```python
from build123d import *

# Parameters (mm, degrees)
ESQUISSE1_W        = 12.8
ESQUISSE1_H        = 9
BOSS_EXTRU_1_DEPTH = 6.8
ESQUISSE2_W        = 1
ESQUISSE2_H        = 2
BOSS_EXTRU_2_DEPTH = 4
ESQUISSE3_R        = 3
BOSS_EXTRU_3_DEPTH = 9
ESQUISSE4_R        = 1.5
BOSS_EXTRU_4_DEPTH = 10


with BuildPart() as part:
    # Esquisse1 → Boss.-Extru.1 (new body)
    with BuildSketch(Plane.XY):
        with Locations((6.4, 4.5)):
            Rectangle(ESQUISSE1_W, ESQUISSE1_H)
    extrude(amount=BOSS_EXTRU_1_DEPTH)

    # Esquisse2 → Boss.-Extru.2 (add)
    with BuildSketch(Plane.XZ):
        with Locations((1.4, 2.9)):
            Rectangle(ESQUISSE2_W, ESQUISSE2_H)
        with Locations((6.4, 2.9)):
            Rectangle(ESQUISSE2_W, ESQUISSE2_H)
        with Locations((11.4, 2.9)):
            Rectangle(ESQUISSE2_W, ESQUISSE2_H)
    extrude(amount=BOSS_EXTRU_2_DEPTH)

    # Esquisse3 → Boss.-Extru.3 (add)
    with BuildSketch(Plane(origin=(0, 9, 0), x_dir=(1, 0, 0), z_dir=(0, 1, 0))):
        with Locations((6.4, -3.4)):
            Circle(ESQUISSE3_R)
    extrude(amount=BOSS_EXTRU_3_DEPTH)

    # Esquisse4 → Boss.-Extru.4 (add)
    with BuildSketch(Plane(origin=(0, 18, 0), x_dir=(1, 0, 0), z_dir=(0, 1, 0))):
        with Locations((6.4, -3.4)):
            Circle(ESQUISSE4_R)
    extrude(amount=BOSS_EXTRU_4_DEPTH)


solid = part.part
```
Source: CAD feature listing. Evaluate the final solid. Frame: model axes, mm. A direction names the side the tool comes from. Round coordinates to 2 decimals unless told otherwise and drop trailing zeros. Loops run counter-clockwise (first coordinate to the right, second up) from the corner with the lowest first, then second, coordinate; pieces in that order, holes last.
1. Mould query, pull axis X, two halves, no side actions, for faces 6 (the flat face through (1.4, -2, 1.9)), 7 (the cylindrical face through (3.4, 13.4, 3.3)), 8 (the flat face through (6.3, 0, 4.1)). Classes: released by +X, released by -X, zero draft, split by the parting line, or undercut.
2. Section query C-C on y = 13. Output: boundary loops of the cut face in (x, z), and give its area (3 significant figures).
3. Section query D-D on x = 6.4. Output: boundary loops of the cut face in (y, z).
4. Access query for faces 1 (the flat face through (0.9, -2, 3)), 2 (the flat face through (5.9, -2, 3)), 3 (the flat face through (3, 9, 3)), 4 (the flat face through (6.4, -2, 1.9)), 5 (the flat face through (1.4, -2, 3.9)). Directions: +Z, -Z, +X, -X, +Y, -Y. A direction counts if a zero-diameter tool reaches every point of the face in a straight line with its end or side. Return the directions, or none.
5. Contact query for flat-ended pins moving along their axis: pin 1 (0.5 mm diameter, centred on x = 11.5, y = -1.5, fed in from -Z); pin 2 (3 mm diameter, centred on y = 20.5, z = 3.5, fed in from +X); pin 3 (2 mm diameter, centred on y = -2, z = 3, fed in from +X). Output: stop coordinate, or through.
6. Section query A-A on x = 4. Output: boundary loops of the cut face in (y, z).
7. Section query B-B on z = 3.4. Output: boundary loops of the cut face in (x, y), and give its area (3 significant figures).
8. Ray query, L1, parallel to X at y = -2, z = 2; L2, parallel to Y at x = 4, z = 6; L3, parallel to Y at x = 7.75, z = 4.75. Return the intervals inside material, ascending.
Answers below:
1. face 6: zero draft
1. face 7: split by the parting line
1. face 8: undercut
2. outline: circle Ø6 at (6.4, 3.4)
2. area: 28.3 mm2
3. outline: (-4, 1.9) - (0, 1.9) - (0, 0) - (9, 0) - (9, 0.4) - (18, 0.4) - (18, 1.9) - (28, 1.9) - (28, 4.9) - (18, 4.9) - (18, 6.4) - (9, 6.4) - (9, 6.8) - (0, 6.8) - (0, 3.9) - (-4, 3.9) - close
4. face 1: +Z, -Z, -X, -Y
4. face 2: +Z, -Z, -Y
4. face 3: +Y
4. face 4: -Z, +X, -X, -Y
4. face 5: +Z, +X, -X, -Y
5. pin 1: stops at z = 1.9
5. pin 2: stops at x = 7.9
5. pin 3: stops at x = 11.9
6. outline: (0, 0) - (9, 0) - (9, 1.6) - (18, 1.6) - (18, 5.2) - (9, 5.2) - (9, 6.8) - (0, 6.8) - close
7. outline: (0, 0) - (0.9, 0) - (0.9, -4) - (1.9, -4) - (1.9, 0) - (5.9, 0) - (5.9, -4) - (6.9, -4) - (6.9, 0) - (10.9, 0) - (10.9, -4) - (11.9, -4) - (11.9, 0) - (12.8, 0) - (12.8, 9) - (9.4, 9) - (9.4, 18) - (7.9, 18) - (7.9, 28) - (4.9, 28) - (4.9, 18) - (3.4, 18) - (3.4, 9) - (0, 9) - close
7. area: 211 mm2
8. L1: x = 0.9 to 1.9, 5.9 to 6.9, 10.9 to 11.9
8. L2: y = 0 to 9
8. L3: y = 0 to 18
